from build123d import *

# Parameters (mm, degrees)
F0_W     = 196.85
F0_H     = 88.9
F1_DEPTH = 9.525
F3_DEPTH = 25.4
F4_W     = 19.05
F4_H     = 87.3125
F5_DEPTH = 4.7625


# Not quite as in the source:
# - a length typed as a fraction of an inch, garbled in the dataset ("3 / 203.2 mm" for 3/8 in), is restored


with BuildPart() as f1:
    # F0 (on Top) → F1 (new body)
    with BuildSketch(Plane.XY):
        with Locations((98.425, 44.45)):
            Rectangle(F0_W, F0_H)
    extrude(amount=F1_DEPTH)

    # F2 (on face) → F3 (cut)
    with BuildSketch(Plane.XY.offset(9.525)):
        with BuildLine():
            ThreePointArc((17.4625, 12.7), (15.08125, 15.08125), (12.7, 12.7))
            Line((12.7, 12.7), (17.4625, 12.7))
        make_face()
        with BuildLine():
            Line((12.7, 76.2), (12.7, 12.7))
            ThreePointArc((12.7, 12.7), (15.08125, 15.08125), (17.4625, 12.7))
            Line((17.4625, 12.7), (17.4625, 76.2))
            ThreePointArc((17.4625, 76.2), (15.08125, 73.81875), (12.7, 76.2))
        make_face()
        with BuildLine():
            Line((17.4625, 12.7), (12.7, 12.7))
            ThreePointArc((12.7, 12.7), (15.08125, 10.31875), (17.4625, 12.7))
        make_face()
        with BuildLine():
            ThreePointArc((17.4625, 76.2), (15.08125, 78.58125), (12.7, 76.2))
            Line((12.7, 76.2), (17.4625, 76.2))
        make_face()
        with BuildLine():
            Line((17.4625, 76.2), (12.7, 76.2))
            ThreePointArc((12.7, 76.2), (15.08125, 73.81875), (17.4625, 76.2))
        make_face()
        with BuildLine():
            ThreePointArc((179.3875, 12.7), (181.76875, 10.31875), (184.15, 12.7))
            Line((184.15, 12.7), (179.3875, 12.7))
        make_face()
        with BuildLine():
            ThreePointArc((179.3875, 12.7), (181.76875, 15.08125), (184.15, 12.7))
            Line((184.15, 12.7), (184.15, 76.2))
            ThreePointArc((184.15, 76.2), (181.76875, 73.81875), (179.3875, 76.2))
            Line((179.3875, 76.2), (179.3875, 12.7))
        make_face()
        with BuildLine():
            Line((179.3875, 12.7), (184.15, 12.7))
            ThreePointArc((184.15, 12.7), (181.76875, 15.08125), (179.3875, 12.7))
        make_face()
        with BuildLine():
            ThreePointArc((179.3875, 76.2), (181.76875, 73.81875), (184.15, 76.2))
            Line((184.15, 76.2), (179.3875, 76.2))
        make_face()
        with BuildLine():
            Line((179.3875, 76.2), (184.15, 76.2))
            ThreePointArc((184.15, 76.2), (181.76875, 78.58125), (179.3875, 76.2))
        make_face()
        with BuildLine():
            ThreePointArc((34.13125, 73.81875), (33.4337980227, 75.5025480227), (31.75, 76.2))
            Line((31.75, 76.2), (31.75, 71.4375))
            ThreePointArc((31.75, 71.4375), (33.4337980227, 72.1349519773), (34.13125, 73.81875))
        make_face()
        with BuildLine():
            Line((165.1, 76.2), (31.75, 76.2))
            ThreePointArc((31.75, 76.2), (33.4337980227, 75.5025480227), (34.13125, 73.81875))
            ThreePointArc((34.13125, 73.81875), (33.4337980227, 72.1349519773), (31.75, 71.4375))
            Line((31.75, 71.4375), (165.1, 71.4375))
            ThreePointArc((165.1, 71.4375), (162.71875, 73.81875), (165.1, 76.2))
        make_face()
        with BuildLine():
            Line((31.75, 71.4375), (31.75, 76.2))
            ThreePointArc((31.75, 76.2), (29.36875, 73.81875), (31.75, 71.4375))
        make_face()
        with BuildLine():
            ThreePointArc((167.48125, 73.81875), (166.7837980227, 75.5025480227), (165.1, 76.2))
            Line((165.1, 76.2), (165.1, 71.4375))
            ThreePointArc((165.1, 71.4375), (166.7837980227, 72.1349519773), (167.48125, 73.81875))
        make_face()
        with BuildLine():
            Line((165.1, 71.4375), (165.1, 76.2))
            ThreePointArc((165.1, 76.2), (162.71875, 73.81875), (165.1, 71.4375))
        make_face()
        with BuildLine():
            ThreePointArc((34.13125, 15.08125), (33.4337980227, 16.7650480227), (31.75, 17.4625))
            Line((31.75, 17.4625), (31.75, 12.7))
            ThreePointArc((31.75, 12.7), (33.4337980227, 13.3974519773), (34.13125, 15.08125))
        make_face()
        with BuildLine():
            Line((165.1, 17.4625), (31.75, 17.4625))
            ThreePointArc((31.75, 17.4625), (33.4337980227, 16.7650480227), (34.13125, 15.08125))
            ThreePointArc((34.13125, 15.08125), (33.4337980227, 13.3974519773), (31.75, 12.7))
            Line((31.75, 12.7), (165.1, 12.7))
            ThreePointArc((165.1, 12.7), (162.71875, 15.08125), (165.1, 17.4625))
        make_face()
        with BuildLine():
            Line((31.75, 12.7), (31.75, 17.4625))
            ThreePointArc((31.75, 17.4625), (29.36875, 15.08125), (31.75, 12.7))
        make_face()
        with BuildLine():
            ThreePointArc((167.48125, 15.08125), (166.7837980227, 16.7650480227), (165.1, 17.4625))
            Line((165.1, 17.4625), (165.1, 12.7))
            ThreePointArc((165.1, 12.7), (166.7837980227, 13.3974519773), (167.48125, 15.08125))
        make_face()
        with BuildLine():
            Line((165.1, 12.7), (165.1, 17.4625))
            ThreePointArc((165.1, 17.4625), (162.71875, 15.08125), (165.1, 12.7))
        make_face()
    extrude(amount=-F3_DEPTH, mode=Mode.SUBTRACT)

    # F4 (on face) → F5 (cut)
    with BuildSketch(Plane.XY.offset(9.525)):
        with Locations((15.08125, 44.45)):
            Rectangle(F4_W, F4_H)
        with Locations((181.76875, 44.45)):
            Rectangle(F4_W, F4_H)
    extrude(amount=-F5_DEPTH, mode=Mode.SUBTRACT)


solid = f1.part
Geometry: final body of the model. Coordinates: model frame, mm. A direction names the side the tool comes from. Coordinates: 2 decimals unless noted, no trailing zeros. Loops run counter-clockwise (first coordinate to the right, second up) from the corner with the lowest first, then second, coordinate; pieces in that order, holes last. Notation, with made-up numbers: (-9, 25) - (0, 25) arc R21 ccw to (0, 42) - close; hole circle Ø3 at (5.25, 14). An arc over 180 degrees is marked (long way). One line per question, with ' | ' between items. Start each with the question number.
(1) Reachability of faces 1 (the cylindrical face through (181.72, 10.32, 2.41)), 2 (the flat face through (15, 0.794, 7)), 3 (the flat face through (196.85, 44, 5)) from +Z, -Z, +X, -X, +Y, -Y: full face, straight path, thin tool, end or side. Return the list, or none.
(2) First-contact query: pin 1 (9.5 mm diameter, centred on x = 14.5, y = 31.5, fed in from +Z). Flat tip, straight axial feed; report the tip coordinate or a pass-through.
(3) Cut plane D-D on x = 175.5. Output: boundary loops of the cut face in (y, z) (1 decimal).
(4) Cut plane B-B on x = 49. Output: boundary loops of the cut face in (y, z) (1 decimal), and give its area (3 significant figures).
(5) Cut plane A-A on y = 49. Count the separate pieces of the cut face and the enclosed holes in it, and give its area (3 significant figures).
(6) Cut plane C-C on z = 3.25. Output: boundary loops of the cut face in (x, y).
(7) Draft query along Y for faces 4 (the flat face through (97, 0, 5)), 5 (the flat face through (12.7, 45, 2)), 6 (the flat face through (97, 45, 9.525)), 7 (the flat face through (172.244, 44, 7)). Return one class per face: +Y half, -Y half, draft (parallel to the pull), parting line (faces both ways), or undercut.
(8) Ray query, L1, parallel to X at y = 19, z = 2; L2, parallel to Y at x = 68, z = 3.75; L3, parallel to X at y = 41, z = 5.5. Return the intervals inside material, ascending. Write a range as from..to.
Here are the results:
1) face 1: +Z, -Z | face 2: +Z | face 3: +Z, -Z, +X, +Y, -Y
2) pin 1: z = 4.76
3) outline: (0, 0) - (88.9, 0) - (88.9, 9.5) - (88.1, 9.5) - (88.1, 4.8) - (0.8, 4.8) - (0.8, 9.5) - (0, 9.5) - close
4) outline: (0, 0) - (12.7, 0) - (12.7, 9.5) - (0, 9.5) - close; (17.5, 0) - (71.4, 0) - (71.4, 9.5) - (17.5, 9.5) - close; (76.2, 0) - (88.9, 0) - (88.9, 9.5) - (76.2, 9.5) - close | area: 756 mm²
5) separate pieces: 3 | enclosed holes: 0 | area: 1,650 mm²
6) outline: (0, 0) - (196.85, 0) - (196.85, 88.9) - (0, 88.9) - close; hole (12.7, 12.7) arc R2.38 ccw to (17.46, 12.7) - (17.46, 76.2) arc R2.38 ccw to (12.7, 76.2) - close; hole (31.75, 12.7) - (165.1, 12.7) arc R2.38 ccw to (165.1, 17.46) - (31.75, 17.46) arc R2.38 ccw to start; hole (31.75, 71.44) - (165.1, 71.44) arc R2.38 ccw to (165.1, 76.2) - (31.75, 76.2) arc R2.38 ccw to start; hole (179.39, 12.7) arc R2.38 ccw to (184.15, 12.7) - (184.15, 76.2) arc R2.38 ccw to (179.39, 76.2) - close
7) face 4: -Y half | face 5: undercut | face 6: draft | face 7: undercut
8) L1: 0..12.7, 17.46..179.39, 184.15..196.85 | L2: 0..12.7, 17.46..71.44, 76.2..88.9 | L3: 0..5.56, 24.61..172.24, 191.29..196.85
